from build123d import *

# Parameters (mm, degrees)
BOSS_EXTRUDE1_DEPTH = 25.4
SKETCH5_R           = 2.4892
CUT_EXTRUDE1_DEPTH  = 43.240627659
SKETCH6_R           = 2.4892
CUT_EXTRUDE2_DEPTH  = 43.240627659


with BuildPart() as part:
    # Sketch2 → Boss-Extrude1 (new body)
    with BuildSketch(Plane.XY):
        Polygon((0, 0), (0, -25.4), (3.175, -25.4), (3.175, -3.175), (25.4, -3.175), (25.4, 0), align=None)
    extrude(amount=BOSS_EXTRUDE1_DEPTH)

    # Sketch5 → Cut-Extrude1 (cut, through all)
    with BuildSketch(Plane(origin=(3.175, 0, 0), x_dir=(0, 0, -1), z_dir=(1, 0, 0))):
        with Locations(Location((-6.35, -12.7, 0), (0, 0, 90))):
            Circle(SKETCH5_R)
        with Locations(Location((-19.05, -12.7, 0), (0, 0, 90))):
            Circle(SKETCH5_R)
        with Locations((-31.75, -12.7)):
            Circle(SKETCH5_R)
        with Locations((-44.45, -12.7)):
            Circle(SKETCH5_R)
    extrude(amount=-CUT_EXTRUDE1_DEPTH, mode=Mode.SUBTRACT)

    # Sketch6 → Cut-Extrude2 (cut, through all)
    with BuildSketch(Plane.XZ.offset(3.175)):
        with Locations((12.7, 6.35)):
            Circle(SKETCH6_R)
        with Locations((12.7, 19.05)):
            Circle(SKETCH6_R)
        with Locations((12.7, 31.75)):
            Circle(SKETCH6_R)
        with Locations((12.7, 44.45)):
            Circle(SKETCH6_R)
    extrude(amount=-CUT_EXTRUDE2_DEPTH, mode=Mode.SUBTRACT)


solid = part.part
Here's how the part is built. I have some questions about the finished solid (model axes, mm). A direction names the side the tool comes from. Round coordinates to 2 decimals unless told otherwise and drop trailing zeros. Order: outer loops, then holes, each group sorted by start corner. A loop starts at its lowest first (then second) coordinate and runs counter-clockwise, first axis right, second up. Notation, with made-up numbers: (45, 34.25) -> (71, 34.25) arc R20 ccw to (71, 60.25) -> close; hole circle Ø1 at (39.5, 39). An arc over 180 degrees is marked (long way). Return JSON: item names as keys, results as strings.
Q1. If we section it at C-C on x = 12.7: List the corners of the cut face in (y, z) for me (3 decimals).
Filled sheet:
{"outline": "(-3.175, 0) -> (0, 0) -> (0, 3.861) -> (-3.175, 3.861) -> close; (-3.175, 8.839) -> (0, 8.839) -> (0, 16.561) -> (-3.175, 16.561) -> close; (-3.175, 21.539) -> (0, 21.539) -> (0, 25.4) -> (-3.175, 25.4) -> close"}
Q2. If we mould it in two halves opening along Z, with no side actions, what happens to faces 3 (the flat face through (2, -7, 0)), 4 (the flat face through (14, -3.175, 13)), 5 (the cylindrical face through (1.61, -13.24, 16.62))? For each: released by +Z, released by -Z, zero draft, split by the parting line, or undercut.
Filled sheet:
{"face 3": "released by -Z", "face 4": "zero draft", "face 5": "undercut"}
Q3. If we section it at B-B on y = -12.7: List the corners of the cut face in (x, z) for me (3 decimals).
Filled sheet:
{"outline": "(0, 0) -> (3.175, 0) -> (3.175, 3.861) -> (0, 3.861) -> close; (0, 8.839) -> (3.175, 8.839) -> (3.175, 16.561) -> (0, 16.561) -> close; (0, 21.539) -> (3.175, 21.539) -> (3.175, 25.4) -> (0, 25.4) -> close"}
Q4. Which directions (+Z, -Z, +X, -X, +Y, -Y) give clear straight access to the entire face, cutting with the end or side of a thin tool? Please do faces 1 (the flat face through (25.4, -2, 13)), 2 (the flat face through (3.175, -14, 13)).
Filled sheet:
{"face 1": "+Z, -Z, +X, +Y, -Y", "face 2": "+Z, -Z, +X, -Y"}
Q5. I need wall thicknesses on line 1 along Z through (x, y) = (12.7, -1.5); line 2 along Y through (x, z) = (7, 13.75) (3 decimals); line 3 along X through (y, z) = (-18, 1) (3 decimals). Which ranges of each line are inside material? Lowest first, please. Write a range as from..to.
Filled sheet:
{"line 1": "z = 0..3.86, 8.84..16.56, 21.54..25.4", "line 2": "y = -3.175..0", "line 3": "x = 0..3.175"}
Q6. For pin 1 Ø3 at (y, z) = (-6, 5.5) entering from +X (3 decimals); pin 2 Ø12 at (x, y) = (12.5, -11) entering from +Z; pin 3 Ø3 at (x, z) = (17.5, 15) entering from -Y (3 decimals), each with a flat end and sliding along its axis, tell me the tip position at first contact or that it passes through.
Filled sheet:
{"pin 1": "stops at x = 3.175", "pin 2": "passes through", "pin 3": "stops at y = -3.175"}
Q7. If we section it at A-A on z = 6.35: List the corners of the cut face in (x, y) for me (3 decimals), plus the area to 3 significant figures.
Filled sheet:
{"outline": "(0, -25.4) -> (3.175, -25.4) -> (3.175, -15.189) -> (0, -15.189) -> close; (0, -10.211) -> (3.175, -10.211) -> (3.175, -3.175) -> (10.211, -3.175) -> (10.211, 0) -> (0, 0) -> close; (15.189, -3.175) -> (25.4, -3.175) -> (25.4, 0) -> (15.189, 0) -> close", "area": "120 mm^2"}
Q8. If we section it at D-D on z = 9.5: List the corners of the cut face in (x, y) for me (3 decimals), plus the area to 3 significant figures.
Filled sheet:
{"outline": "(0, -25.4) -> (3.175, -25.4) -> (3.175, -3.175) -> (25.4, -3.175) -> (25.4, 0) -> (0, 0) -> close", "area": "151 mm^2"}
